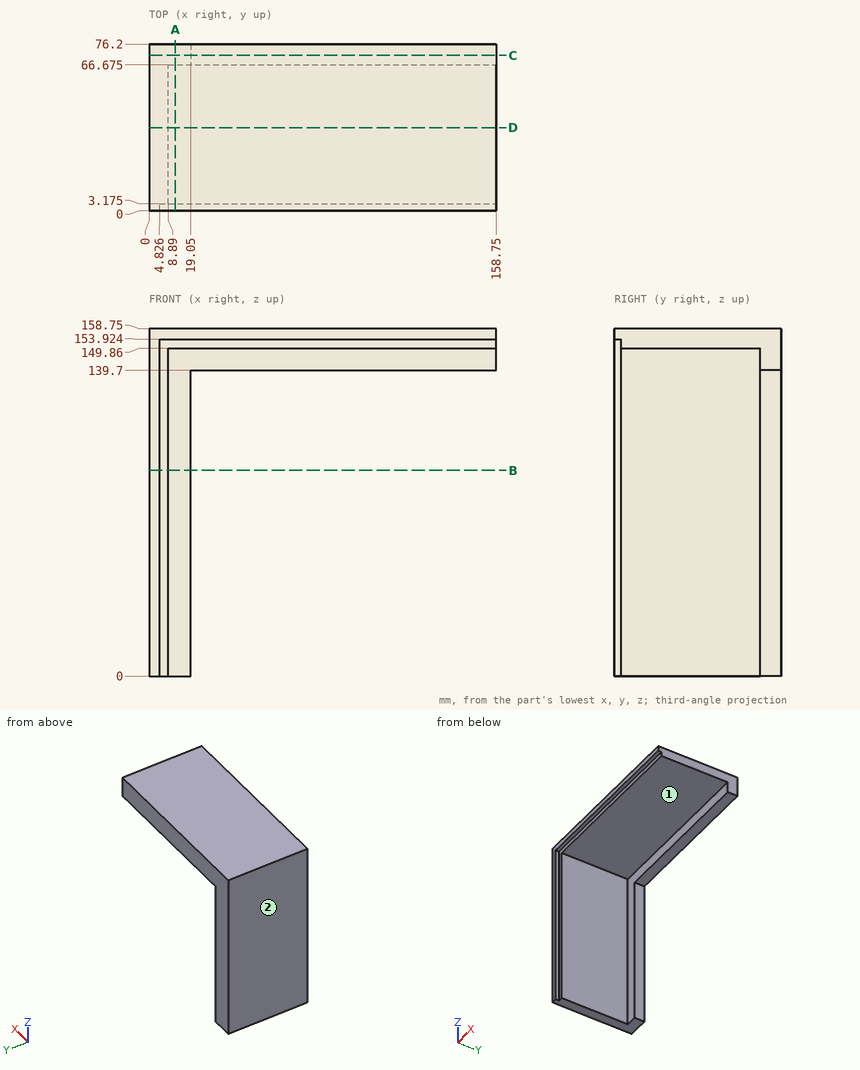
Geometry: see drawing. Coordinates: mm, zero at the bounding-box minimum. A direction names the side the tool comes from. Give positions to 0.01 mm unless a question says otherwise; leave off trailing zeros. Write each loop counter-clockwise with the first axis right and the second up, starting at its lowest first coordinate (ties: lowest second). Pieces come first, ordered by that corner, then holes. Notation, with made-up numbers: M 76.5,-37.5 L 130.5,-37.5 A18 ccw 130.5,-17.5 Z; hole C -30,-19 d11. An arc over 180 degrees is marked long. Answer in a Markdown table with one row per item. Add a question column.
(1) Section D-D on y = 38. Return loops of the section in (x, z), and give its area (3 significant figures).
(2) Section B-B on z = 94. Return loops of the section in (x, y) (3 decimals), and give its area (3 significant figures).
(3) First-contact query: pin 1 (10.5 mm diameter, centred on y = 72.5, z = 73, fed in from +X); pin 2 (3 mm diameter, centred on x = 17.5, z = 112.5, fed in from -Y) (3 decimals); pin 3 (10 mm diameter, centred on y = 61, z = 85, fed in from +X). Flat tips, straight axial feed; report the tip coordinate or a pass-through.
(4) Reachability of the marked faces 1 and 2 from +Z, -Z, +X, -X, +Y, -Y: full face, straight path, thin tool, end or side. Return the list, or none.
(5) Section A-A on x = 12. Return loops of the section in (y, z) (3 decimals), and give its area (3 significant figures).
(6) Section C-C on y = 71. Return loops of the section in (x, z), and give its area (3 significant figures).
(7) Ray query, line 1 (X direction, y = 24.5, z = 81); line 2 (Z direction, x = 40.5, y = 43); line 3 (Y direction, x = 12.5, z = 127.5) (3 decimals). Return the intervals inside material, ascending.
Result set:
| question | item | result |
|---|---|---|
| 1 | outline | M 0,0 L 8.89,0 L 8.89,149.86 L 158.75,149.86 L 158.75,158.75 L 0,158.75 Z |
| 1 | area | 2,740 mm^2 |
| 2 | outline | M 0,0 L 4.826,0 L 4.826,3.175 L 8.89,3.175 L 8.89,66.675 L 19.05,66.675 L 19.05,76.2 L 0,76.2 Z |
| 2 | area | 761 mm^2 |
| 3 | pin 1 | stops at x = 19.05 |
| 3 | pin 2 | stops at y = 66.675 |
| 3 | pin 3 | stops at x = 8.89 |
| 4 | face 1 | -Z, +X, -Y |
| 4 | face 2 | +Z, -Z, -X, +Y, -Y |
| 5 | outline | M 0,153.924 L 3.175,153.924 L 3.175,149.86 L 66.675,149.86 L 66.675,0 L 76.2,0 L 76.2,158.75 L 0,158.75 Z |
| 5 | area | 2,090 mm^2 |
| 6 | outline | M 0,0 L 19.05,0 L 19.05,139.7 L 158.75,139.7 L 158.75,158.75 L 0,158.75 Z |
| 6 | area | 5,690 mm^2 |
| 7 | line 1 | x = 0 to 8.89 |
| 7 | line 2 | z = 149.86 to 158.75 |
| 7 | line 3 | y = 66.675 to 76.2 |
